Model file for the job. Use its own axes, mm. A direction names the side the tool comes from. Round coordinates to 2 decimals unless told otherwise and drop trailing zeros. Write each loop counter-clockwise with the first axis right and the second up, starting at its lowest first coordinate (ties: lowest second). Pieces come first, ordered by that corner, then holes.
```python
from build123d import *

# Parameters (mm, degrees)
F1_DEPTH  = 22
F3_D      = 3.3
F3_DEPTH  = 3
F3_TIP    = 0.9914200214
F4_R      = 1.5
F5_R      = 5
F7_D      = 3.3
F7_DEPTH  = 3
F7_TIP    = 0.9914200214
F9_D      = 3.3
F9_DEPTH  = 3
F9_TIP    = 0.9914200214
F11_D     = 3.3
F11_DEPTH = 63
F11_TIP   = 0.9914200214


with BuildPart() as f1:
    # F0 (on Top) → F1 (new body)
    with BuildSketch(Plane.XY):
        Polygon((-28.5, -20), (-28.5, 20), (28.5, 20), (28.5, -20), (30.5, -20), (30.5, 18), (63.8553390593, -15.3553390593), (65.8553390593, -13.3553390593), (30.5, 22), (-30.5, 22), (-65.8553390593, -13.3553390593), (-63.8553390593, -15.3553390593), (-30.5, 18), (-30.5, -20), align=None)
    extrude(amount=F1_DEPTH)

    # F3
    with Locations(Plane(origin=(26.25, 26.25, 0), x_dir=(-0.7071067812, 0.7071067812, 0), z_dir=(0.7071067812, 0.7071067812, 0))):
        with Locations((-17.5104076401, 7.5), (-49.5104076401, 7.5)):
            Hole(F3_D / 2, depth=F3_DEPTH)
            with Locations((0, 0, -(F3_DEPTH + F3_TIP / 2))):  # 118° drill point
                Cone(0, F3_D / 2, F3_TIP, mode=Mode.SUBTRACT)

    # F4
    f4_edges = [f1.edges().sort_by_distance(p)[0] for p in [
        (-30.5, 18, 11),
        (30.5, 18, 11),
    ]]
    fillet(f4_edges, radius=F4_R)

    # F5
    f5_edges = [f1.edges().sort_by_distance(p)[0] for p in [
        (-28.5, 20, 11),
        (28.5, 20, 11),
    ]]
    fillet(f5_edges, radius=F5_R)

    # F7
    with Locations(Plane(origin=(-26.25, 26.25, 0), x_dir=(-0.7071067812, -0.7071067812, 0), z_dir=(-0.7071067812, 0.7071067812, 0))):
        with Locations((17.5104076401, 7.5), (49.5104076401, 7.5)):
            Hole(F7_D / 2, depth=F7_DEPTH)
            with Locations((0, 0, -(F7_DEPTH + F7_TIP / 2))):  # 118° drill point
                Cone(0, F7_D / 2, F7_TIP, mode=Mode.SUBTRACT)

    # F9
    with Locations(Plane(origin=(0, 22, 0), x_dir=(-1, 0, 0), z_dir=(0, 1, 0))):
        with Locations((-16, 7.5), (16, 7.5)):
            Hole(F9_D / 2, depth=F9_DEPTH)
            with Locations((0, 0, -(F9_DEPTH + F9_TIP / 2))):  # 118° drill point
                Cone(0, F9_D / 2, F9_TIP, mode=Mode.SUBTRACT)

    # F11 (one way)
    with BuildSketch(Plane(origin=(-30.5, 0, 0), x_dir=(0, -1, 0), z_dir=(-1, 0, 0))):
        with Locations((16, 19), (16, 3)):
            Circle(F11_D / 2)
    extrude(amount=-F11_DEPTH, mode=Mode.SUBTRACT)
    with Locations(Plane(origin=(-30.5, 0, 0), x_dir=(0, -1, 0), z_dir=(-1, 0, 0))):
        with Locations((16, 19), (16, 3)):
            with Locations((0, 0, -(F11_DEPTH + F11_TIP / 2))):  # 118° drill point
                Cone(0, F11_D / 2, F11_TIP, mode=Mode.SUBTRACT)


solid = f1.part
```
1) Flat gauge pins, fed straight in: pin 1 Ø2 at (x, y) = (27, -14) entering from -Z; pin 2 Ø6.5 at (x, z) = (-1.5, 12) entering from -Y; pin 3 Ø4 at (y, z) = (-16, 19) entering from -X; pin 4 Ø10 at (y, z) = (-9, 10) entering from +X. Where does each tip first touch, or does it go through?
2) Cut at B-B on x = 16. List the corners of the cut face in (y, z), and give its area (3 significant figures).
3) Wall check: probe 1 along Z at (x, y) = (29.15, -16); probe 2 along X at (y, z) = (-10, 13.25); probe 3 along X at (y, z) = (-5.5, 6.75). Give the ranges that are in metal, low to high.
4) Cut at A-A on y = -5.5. List the corners of the cut face in (x, z), and give its area (3 significant figures).
5) Cut at D-D on x = -50. List the corners of the cut face in (y, z), and give its area (3 significant figures).
6) Cut at C-C on z = 12. List the corners of the cut face in (x, y).
7) Which spindle directions (+Z, -Z, +X, -X, +Y, -Y) get a long thin tool onto all of the face, cutting with end or side? Do faces 5 (the face through (-29.514, -17.574, 3.496)), 6 (the face through (-47.9, 4.6, 10.8)), 7 (the face through (-30.5, -3, 11)). Say none if no direction does.
8) Pull direction Z, two halves, no side cores. Call faces 1 (the face through (48.4, 4.1, 10.8)), 2 (the face through (0, 21, 22)), 3 (the face through (61.358, -10.886, 7.996)), 4 (the face through (-59.132, -8.66, 7.996)): released by +Z, released by -Z, zero draft, split by the parting line, or undercut.
Result sheet:
1. pin 1: passes through
1. pin 2: stops at y = 20
1. pin 3: stops at x = -65.21
1. pin 4: stops at x = 65.86
2. outline: (20, 0) - (22, 0) - (22, 5.85) - (20, 5.85) - close; (20, 9.15) - (22, 9.15) - (22, 22) - (20, 22) - close
2. area: 37.4 mm2
3. probe 1: z = 0 to 1.35, 4.65 to 17.35, 20.65 to 22
3. probe 2: x = -62.5 to -58.5, -30.5 to -28.5, 28.5 to 30.5, 58.5 to 62.5
3. probe 3: x = -58 to -54, -30.5 to -28.5, 28.5 to 30.5, 54 to 58
4. outline: (-58, 0) - (-54, 0) - (-54, 22) - (-58, 22) - close; (-30.5, 0) - (-28.5, 0) - (-28.5, 22) - (-30.5, 22) - close; (28.5, 0) - (30.5, 0) - (30.5, 22) - (28.5, 22) - close; (54, 0) - (58, 0) - (58, 22) - (54, 22) - close
4. area: 264 mm2
5. outline: (-1.5, 0) - (2.5, 0) - (2.5, 22) - (-1.5, 22) - close
5. area: 88.0 mm2
6. outline: (-65.86, -13.36) - (-63.86, -15.36) - (-33.06, 15.44) arc R1.5 cw to (-30.5, 14.38) - (-30.5, -20) - (-28.5, -20) - (-28.5, 15) arc R5 cw to (-23.5, 20) - (23.5, 20) arc R5 cw to (28.5, 15) - (28.5, -20) - (30.5, -20) - (30.5, 14.38) arc R1.5 cw to (33.06, 15.44) - (63.86, -15.36) - (65.86, -13.36) - (30.5, 22) - (-30.5, 22) - close
7. face 5: none
7. face 6: +Z, -Z, -X, +Y
7. face 7: +Z, -Z, -Y
8. face 1: zero draft
8. face 2: released by +Z
8. face 3: undercut
8. face 4: undercut
